Geometry: see drawing. Coordinates: mm, zero at the bounding-box minimum. Coordinates: 2 decimals unless noted, no trailing zeros. Write each loop counter-clockwise with the first axis right and the second up, starting at its lowest first coordinate (ties: lowest second). Pieces come first, ordered by that corner, then holes. Notation, with made-up numbers: (54.5, 49.25) - (60.5, 49.25) arc R24 ccw to (60.5, 87.25) - close; hole circle Ø6 at (61, 11.25). An arc over 180 degrees is marked (long way). One line per question, with ' | ' between items. Start each with the question number.
1) Section query D-D on x = 32.5. Return loops of the section in (y, z).
2) Section query A-A on z = 8. Return loops of the section in (x, y) (1 decimal), and give its area (3 significant figures).
3) Section query C-C on x = 50.8. Return loops of the section in (y, z) (1 decimal), and give its area (3 significant figures).
4) Section query B-B on y = 25.4. Return loops of the section in (x, z) (1 decimal), and give its area (3 significant figures).
5) Line query: line 1 (Y direction, x = 50.8, z = 12.75) (1 decimal); line 2 (X direction, y = 25.4, z = 7.75) (1 decimal); line 3 (Z direction, x = 53, y = 20). Output: solid intervals per line, ascending.
6) Draft query along Y for the marked faces 1, 2, 3 and 4. Return one class per face: released by +Y, released by -Y, zero draft, split by the parting line, or undercut.
7) First-contact query: P1, Ø5, axis at x = 26, y = 22.5, coming from the -Z side; P2, Ø5, axis at x = 50.8, y = 25.4, coming from the -Z side; P3, Ø1.5, axis at x = 59.5, y = 19.5, coming from the -Z side; P4, Ø2, axis at x = 31.5, y = 13.5, coming from the -Z side. Flat tips, straight axial feed; report the tip coordinate or a pass-through.
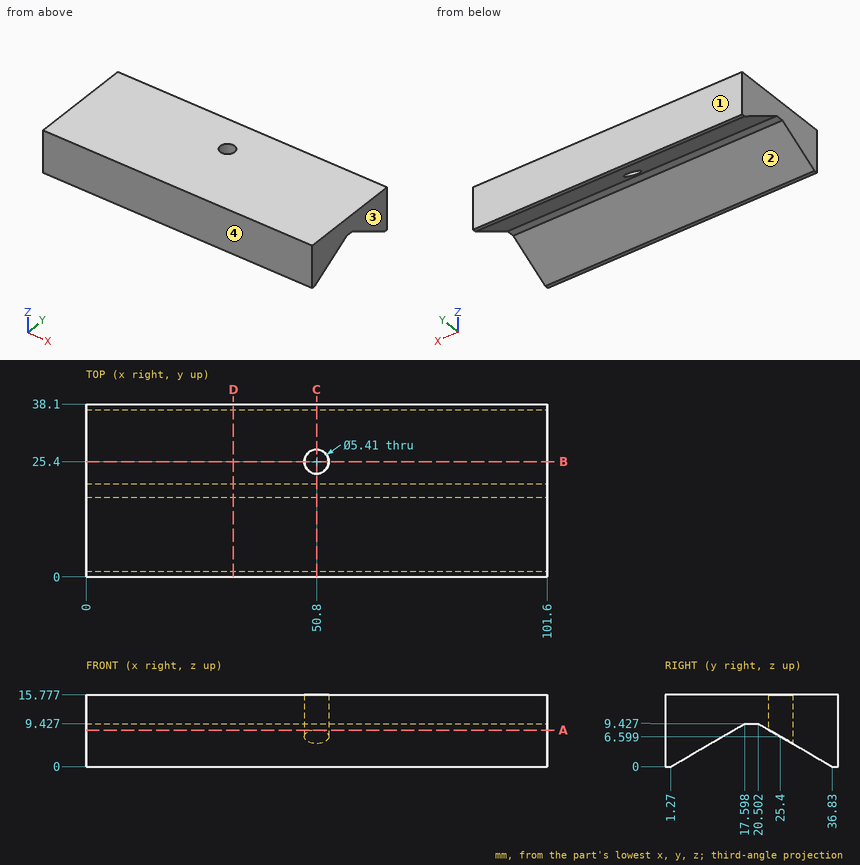
Answer key:
1) outline: (0, 0) - (1.27, 0) - (17.6, 9.43) - (20.5, 9.43) - (36.83, 0) - (38.1, 0) - (38.1, 15.78) - (0, 15.78) - close
2) outline: (0, 0) - (101.6, 0) - (101.6, 15.1) - (0, 15.1) - close; (0, 23) - (49.6, 23) arc R2.7 cw (long way) to (52, 23) - (101.6, 23) - (101.6, 38.1) - (0, 38.1) - close | area: 3,050 mm²
3) outline: (0, 0) - (1.3, 0) - (17.6, 9.4) - (20.5, 9.4) - (22.7, 8.2) - (22.7, 15.8) - (0, 15.8) - close; (28.1, 5) - (36.8, 0) - (38.1, 0) - (38.1, 15.8) - (28.1, 15.8) - close | area: 370 mm²
4) outline: (0, 6.6) - (48.1, 6.6) - (48.1, 15.8) - (0, 15.8) - close; (53.5, 6.6) - (101.6, 6.6) - (101.6, 15.8) - (53.5, 15.8) - close | area: 883 mm²
5) line 1: 0 to 22.7, 28.1 to 38.1 | line 2: 0 to 48.1, 53.5 to 101.6 | line 3: 9.43 to 15.78
6) face 1: released by +Y | face 2: undercut | face 3: zero draft | face 4: released by -Y
7) P1: z = 6.83 | P2: through | P3: z = 9.43 | P4: z = 6.48
